```python
from build123d import *

# Parameters (mm, degrees)
SKETCH_1_R          = 1.6
EXTRUDE_1_DEPTH     = 10
SKETCH_2_R          = 5
CUT_EXTRUDE_1_DEPTH = 25
SKETCH_3_R          = 3
CUT_EXTRUDE_2_DEPTH = 3
CUT_EXTRUDE_START   = -5
SKETCH_4_R          = 5
SKETCH_4_R_2        = 3.5
CUT_EXTRUDE_3_DEPTH = 5


with BuildPart() as part:
    # 草图1 → 凸台-拉伸1 (new body)
    with BuildSketch(Plane(origin=(0, 0, 0), x_dir=(1, 0, 0), z_dir=(0, 1, 0))):
        with BuildLine():
            Line((20, 0), (50, 0))
            ThreePointArc((50, 0), (64.142135624, 5.857864376), (70, 20))
            Line((70, 20), (70, 50))
            ThreePointArc((70, 50), (64.142135624, 64.142135624), (50, 70))
            Line((50, 70), (20, 70))
            ThreePointArc((20, 70), (5.857864376, 64.142135624), (0, 50))
            Line((0, 50), (0, 20))
            ThreePointArc((0, 20), (5.857864376, 5.857864376), (20, 0))
        make_face()
        with Locations(Location((10, 60, 0), (0, 0, 270))):
            Circle(SKETCH_1_R, mode=Mode.SUBTRACT)
        with Locations(Location((60, 60, 0), (0, 0, 270))):
            Circle(SKETCH_1_R, mode=Mode.SUBTRACT)
        with Locations(Location((60, 10, 0), (0, 0, 270))):
            Circle(SKETCH_1_R, mode=Mode.SUBTRACT)
        with Locations(Location((10, 10, 0), (0, 0, 270))):
            Circle(SKETCH_1_R, mode=Mode.SUBTRACT)
    extrude(amount=EXTRUDE_1_DEPTH)

    # 草图2 → 切除-拉伸1 (cut)
    with BuildSketch(Plane(origin=(0, 10, 0), x_dir=(1, 0, 0), z_dir=(0, 1, 0))):
        with Locations(Location((35, 55, 0), (0, 0, 270))):
            Circle(SKETCH_2_R)
        with Locations(Location((54.021130326, 41.180339888, 0), (0, 0, 270))):
            Circle(SKETCH_2_R)
        with Locations(Location((46.755705046, 18.819660113, 0), (0, 0, 270))):
            Circle(SKETCH_2_R)
        with Locations(Location((23.244294954, 18.819660112, 0), (0, 0, 270))):
            Circle(SKETCH_2_R)
        with Locations(Location((15.978869674, 41.180339887, 0), (0, 0, 270))):
            Circle(SKETCH_2_R)
    extrude(amount=-CUT_EXTRUDE_1_DEPTH, mode=Mode.SUBTRACT)

    # 草图3 → 切除-拉伸2 (cut)
    with BuildSketch(Plane(origin=(0, 10, 0), x_dir=(1, 0, 0), z_dir=(0, 1, 0))):
        with Locations(Location((10, 60, 0), (0, 0, 270))):
            Circle(SKETCH_3_R)
        with Locations(Location((60, 60, 0), (0, 0, 270))):
            Circle(SKETCH_3_R)
        with Locations(Location((60, 10, 0), (0, 0, 270))):
            Circle(SKETCH_3_R)
        with Locations(Location((10, 10, 0), (0, 0, 270))):
            Circle(SKETCH_3_R)
    extrude(amount=-CUT_EXTRUDE_2_DEPTH, mode=Mode.SUBTRACT)

    # 草图4 → 切除-拉伸3 (cut)
    with BuildSketch(Plane.XZ.offset(CUT_EXTRUDE_START)):
        with Locations(Location((15.978869674, -41.180339887, 0), (0, 0, 90))):
            Circle(SKETCH_4_R)
        with Locations(Location((35, -55, 0), (0, 0, 90))):
            Circle(SKETCH_4_R)
        with Locations(Location((54.021130326, -41.180339888, 0), (0, 0, 90))):
            Circle(SKETCH_4_R)
        with Locations(Location((46.755705046, -18.819660113, 0), (0, 0, 90))):
            Circle(SKETCH_4_R)
        with Locations(Location((23.244294954, -18.819660112, 0), (0, 0, 90))):
            Circle(SKETCH_4_R)
        with Locations(Location((35, -35, 0), (0, 0, 270))):
            Circle(SKETCH_4_R_2)
    extrude(amount=CUT_EXTRUDE_3_DEPTH, mode=Mode.SUBTRACT)


solid = part.part
```
Source: CAD feature listing. Evaluate the final solid. Frame: model axes, mm. A direction names the side the tool comes from. Coordinates: 2 decimals unless noted, no trailing zeros. Loops run counter-clockwise (first coordinate to the right, second up) from the corner with the lowest first, then second, coordinate; pieces in that order, holes last. Notation, with made-up numbers: M -10.75,79.25 L 41.25,79.25 A20 ccw 41.25,104.25 Z; hole C -21,-27.75 d8. An arc over 180 degrees is marked long. Use a Markdown table: item, result. Add a question column.
Q1. Material intervals for L1, parallel to X at y = 6.5, z = -41.5; L2, parallel to X at y = 1.5, z = -19; L3, parallel to Z at x = 10, y = 3.25, sorted ascending.
Q2. First-contact query: pin 1 (5.5 mm diameter, centred on x = 10, z = -10, fed in from +Y); pin 2 (9 mm diameter, centred on x = 54.02, z = -41.18, fed in from -Y); pin 3 (1.5 mm diameter, centred on x = 55.5, y = 1, fed in from +Z); pin 4 (1 mm diameter, centred on x = 60.5, y = 9, fed in from -Z). Flat tips, straight axial feed; report the tip coordinate or a pass-through.
Q3. Section query C-C, the plane y = 2. State how many separate pieces and enclosed holes the cut face has, and give its area (3 significant figures).
Q4. Draft query along X for faces 4 (the cylindrical face through (60, 9, -63)), 5 (the flat face through (27, 0, -35)), 6 (the flat face through (0, 5, -35)), 7 (the cylindrical face through (18.363, 5.07, -19.904)). Return one class per face: pulls with the +X half, pulls with the -X half, needs draft (parallel to the pull), parting line crosses it, or undercut.
Q5. Access query for faces 1 (the flat face through (8.7, 7, -58.7)), 2 (the flat face through (35, 5, -35)), 3 (the cylindrical face through (61.35, 3.45, -59.14)). Directions: +Z, -Z, +X, -X, +Y, -Y. A direction counts if a zero-diameter tool reaches every point of the face in a straight line with its end or side. Return the directions, or none.
Q6. Section query D-D, the plane z = -54. Return loops of the section in (x, y), and give its area (3 significant figures).
Q7. Section query B-B, the plane z = -35. Return loops of the section in (x, y), and give its area (3 significant figures).
Q8. Section query A-A, the plane x = 35. Return loops of the section in (y, z), and give its area (3 significant figures).
Result:
| question | item | result |
|---|---|---|
| 1 | L1 | x = 0 to 10.99, 20.97 to 49.03, 59.01 to 70 |
| 1 | L2 | x = 0.03 to 18.25, 28.24 to 41.76, 51.75 to 69.97 |
| 1 | L3 | z = -67.32 to -61.6, -58.4 to -11.6, -8.4 to -2.68 |
| 2 | pin 1 | stops at y = 7 |
| 2 | pin 2 | passes through |
| 2 | pin 3 | stops at z = -0.57 |
| 2 | pin 4 | stops at z = -67.32 |
| 3 | separate pieces | 1 |
| 3 | enclosed holes | 10 |
| 3 | area | 4,090 mm2 |
| 4 | face 4 | undercut |
| 4 | face 5 | needs draft |
| 4 | face 6 | pulls with the -X half |
| 4 | face 7 | undercut |
| 5 | face 1 | +Y |
| 5 | face 2 | -Y |
| 5 | face 3 | +Y, -Y |
| 6 | outline | M 0.4,0 L 30.1,0 L 30.1,10 L 0.4,10 Z; M 39.9,0 L 69.6,0 L 69.6,10 L 39.9,10 Z |
| 6 | area | 594 mm2 |
| 7 | outline | M 0,0 L 31.5,0 L 31.5,5 L 38.5,5 L 38.5,0 L 70,0 L 70,10 L 0,10 Z |
| 7 | area | 665 mm2 |
| 8 | outline | M 0,-70 L 10,-70 L 10,-60 L 0,-60 Z; M 0,-50 L 10,-50 L 10,0 L 0,0 L 0,-31.5 L 5,-31.5 L 5,-38.5 L 0,-38.5 Z |
| 8 | area | 565 mm2 |
